Here's how the part is built. I have some questions about the finished solid (model axes, mm). A direction names the side the tool comes from. Round coordinates to 2 decimals unless told otherwise and drop trailing zeros. Order: outer loops, then holes, each group sorted by start corner. A loop starts at its lowest first (then second) coordinate and runs counter-clockwise, first axis right, second up. Notation, with made-up numbers: M 52.25,65.5 L 65.25,65.5 A11 cw 65.25,84.5 Z; hole C 1,-14 d5. An arc over 180 degrees is marked long. Write item = value, one per line. Start each with the question number.
Item 1: I'm going to push flat-ended pins straight in: P1, Ø5, axis at x = 36.5, y = 22.5, coming from the -Z side; P2, Ø5, axis at y = 11, z = -3.5, coming from the -X side; P3, Ø1.8, axis at x = 6, y = -8, coming from the -Z side; P4, Ø2, axis at y = 10, z = -1.5, coming from the -X side. Where does each tip first touch, or does it pass through?
Item 2: I want a section at D-D, the plane x = 28. List the corners of the cut face in (y, z) for me.
Item 3: We'd pull the mould along X, two halves only. Please class faces 4 (the face through (14.55, 17.619, -2.585)), 5 (the face through (2.73, 21.35, -6.82)), 6 (the face through (1.7, -26.2, 0.2)): pulls with the +X half, pulls with the -X half, needs draft (parallel to the pull), parting line crosses it, or undercut.
Item 4: Please list where these lines run through material, in increasing order: L1, parallel to Y at x = 26.5, z = -7.5; L2, parallel to Y at x = 5.5, z = -7; L3, parallel to Z at x = 39, y = 0.
Item 5: I want a section at A-A, the plane x = 36.5. State how many separate pieces and enclosed holes the cut face has, plus the area to 3 significant figures.
Item 6: I want a section at C-C, the plane y = 13. List the corners of the cut face in (x, z) for me.
Item 7: I want a section at B-B, the plane z = 4.5. List the corners of the cut face in (x, y) for me, plus the area to 3 significant figures.
Item 8: For faces 1 (the face through (22, -28, 0)), 2 (the face through (3.89, -5.97, -6.82)), 3 (the face through (29, -16, -7)), which set-ups out of +Z, -Z, +X, -X, +Y, -Y let a thin tool reach every point of the face, with its end or its side?
Autodesk Inventor part; units mm, degrees
ref_plane "YZ Plane" through (0, 0, 0) normal (1, 0, 0) x (0, 1, 0)
ref_plane "XZ Plane" through (0, 0, 0) normal (0, 1, 0) x (-1, 0, 0)
ref_plane "XY Plane" through (0, 0, 0) normal (0, 0, 1) x (1, 0, 0)
sketch "Sketch1" plane through (0, 0, 0) normal (1, 0, 0) x (0, 1, 0)
  line L0 (-28, 12.25) -> (28, 12.25)
  line L1 (28, 12.25) -> (28, -12.25)
  line L2 (28, -12.25) -> (-28, -12.25)
  line L3 (-28, -12.25) -> (-28, 12.25)
  line L4 (-28, 12.25) -> (28, -12.25) construction
  line L5 (28, 12.25) -> (-28, -12.25) construction
  circle A0 centre (13, -4.5) radius 5
  circle A1 centre (0, 4.5) radius 5
  circle A2 centre (-18, -4.5) radius 5
  circle A3 centre (13, -4.5) radius 3
  circle A4 centre (0, 4.5) radius 3
  circle A5 centre (-18, -4.5) radius 3
  point P0 (0, 0)
  dimension "d2" = 56
  dimension "d3" = 24.5
  dimension "d4" = 10
  dimension "d5" = 4.5
  dimension "d6" = 4.5
  dimension "d7" = 15
  dimension "d8" = 6
  dimension "d27" = 10
extrude "Extrusion1" add sketch "Sketch1" along normal blind 42 contours L0 L1 L2 L3 | A0 | A1 | A2
extrude "Extrusion2" cut sketch "Sketch1" along normal blind 29 contours A0 | A1 | A2
sketch "Sketch2" plane through (0, -28, 12.25) normal (0, 0, 1) x (1, 0, 0)
  circle A0 centre (5.5, 50.5) radius 1.75
  circle A1 centre (36.5, 50.5) radius 1.75
  circle A2 centre (36.5, 19.5) radius 1.75
  circle A3 centre (5.5, 19.5) radius 1.75
  line L0 (0, 56) -> (42, 56)
  line L1 (0, 56) -> (0, 0)
  circle A4 centre (36.5, 50.5) radius 3
  circle A5 centre (5.5, 50.5) radius 3
  circle A6 centre (5.5, 19.5) radius 3
  circle A7 centre (36.5, 19.5) radius 3
  point P0 (0, 28)
  dimension "d11" = 5.5
  dimension "d12" = 5.5
  dimension "d13" = 31
  dimension "d14" = 31
  dimension "d15" = 3.5
  dimension "d21" = 6
extrude "Extrusion3" cut sketch "Sketch2" against normal blind 28.75 contours A0 | A1 | A2 | A3
chamfer "Chamfer1" distance 3.5 angle 45 2 edges at (0, 28, 0) (0, -28, 0)
sketch "Sketch3" plane through (42, -28, -12.25) normal (0, 0, -1) x (-1, 0, 0)
  circle A0 centre (5.5, 50.5) radius 3
  circle A1 centre (36.5, 50.5) radius 3
  circle A2 centre (36.5, 19.5) radius 3
  circle A3 centre (5.5, 19.5) radius 3
  point P0 (42, 28)
extrude "Extrusion4" cut sketch "Sketch3" against normal blind 10.5
chamfer "Chamfer2" distance 1.25 angle 45 4 edges at (34.75, 22.5, -1.75) (3.75, 22.5, -1.75) (3.75, -8.5, -1.75) (34.75, -8.5, -1.75)
chamfer "Chamfer3" distance 0.5 angle 45 7 edges at (39.5, 22.5, -12.25) (8.5, 22.5, -12.25) (0, 8, -4.5) (0, -5, 4.5) (0, -23, -4.5) (8.5, -8.5, -12.25) (39.5, -8.5, -12.25)
properties part number "ZaxisMotorMount_3DPrint"
Filled in:
q1.P1 = -1.25
q1.P2 = 29
q1.P3 = through
q1.P4 = 0.26
q2.outline = M -28,-12.25 L 28,-12.25 L 28,12.25 L -28,12.25 Z; hole C -18,-4.5 d10; hole C 0,4.5 d10; hole C 13,-4.5 d10
q3.face_4 = needs draft
q3.face_5 = undercut
q3.face_6 = pulls with the -X half
q4.L1 = -28 to -22, -14 to 9, 17 to 28
q4.L2 = -28 to -22.33, -13.67 to -11.5, -5.5 to 8.67, 17.33 to 19.5, 25.5 to 28
q4.L3 = -12.25 to 1.5, 7.5 to 12.25
q5.separate_pieces = 3
q5.enclosed_holes = 3
q5.area = 1,060 mm^2
q6.outline = M 0,-12.25 L 42,-12.25 L 42,-7.5 L 29,-7.5 L 29,-9.5 L 0.5,-9.5 L 0,-10 Z; M 0,1 L 0.5,0.5 L 29,0.5 L 29,-1.5 L 42,-1.5 L 42,12.25 L 0,12.25 Z
q7.outline = M 0,-24.5 L 3.5,-28 L 42,-28 L 42,-3 L 29,-3 L 29,-5 L 0.5,-5 L 0,-5.5 Z; M 0,5.5 L 0.5,5 L 29,5 L 29,3 L 42,3 L 42,28 L 3.5,28 L 0,24.5 Z; hole C 5.5,-8.5 d3.5; hole C 5.5,22.5 d3.5; hole C 36.5,-8.5 d3.5; hole C 36.5,22.5 d3.5
q7.area = 1,930 mm^2
q8.face_1 = +Z, -Z, +X, -X, -Y
q8.face_2 = -Z
q8.face_3 = -X
